Check sheet for the modelled part. Datum: model origin and axes. Units: mm. Face numbers are marked on the shaded views. Coordinates: 2 decimals unless noted, no trailing zeros. Order: outer loops, then holes, each group sorted by start corner. A loop starts at its lowest first (then second) coordinate and runs counter-clockwise, first axis right, second up.
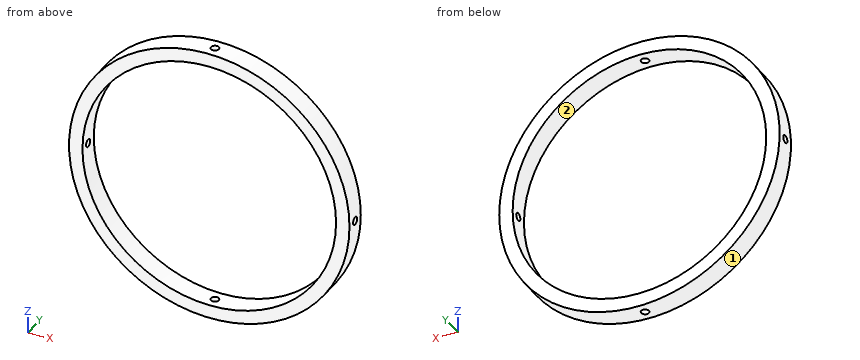
from build123d import *

# Parameters (mm, degrees)
SKETCH1_R               = 52.25
SKETCH1_R_2             = 47.25
BOSS_EXTRUDE1_DEPTH     = 8
SKETCH2_R               = 1.45
CUT_EXTRUDE1_DEPTH      = 53.25
CUT_EXTRUDE1_DEPTH_BACK = 53.25
SKETCH3_R               = 1.45
CUT_EXTRUDE2_DEPTH      = 53.2500001
CUT_EXTRUDE2_DEPTH_BACK = 53.2500001


with BuildPart() as part:
    # Sketch1 → Boss-Extrude1 (new body)
    with BuildSketch(Plane(origin=(0, 0, 0), x_dir=(1, 0, 0), z_dir=(0, 1, 0))):
        Circle(SKETCH1_R)
        Circle(SKETCH1_R_2, mode=Mode.SUBTRACT)
    extrude(amount=BOSS_EXTRUDE1_DEPTH)

    # Sketch2 → Cut-Extrude1 (cut, two sides)
    with BuildSketch(Plane.XY) as cut_extrude1_sk:
        with Locations((0, 4)):
            Circle(SKETCH2_R)
    extrude(amount=CUT_EXTRUDE1_DEPTH, mode=Mode.SUBTRACT)
    extrude(cut_extrude1_sk.sketch, amount=-CUT_EXTRUDE1_DEPTH_BACK, mode=Mode.SUBTRACT)

    # Sketch3 → Cut-Extrude2 (cut, two sides)
    with BuildSketch(Plane(origin=(0, 0, 0), x_dir=(0, 0, -1), z_dir=(1, 0, 0))) as cut_extrude2_sk:
        with Locations((0, 4)):
            Circle(SKETCH3_R)
    extrude(amount=CUT_EXTRUDE2_DEPTH, mode=Mode.SUBTRACT)
    extrude(cut_extrude2_sk.sketch, amount=-CUT_EXTRUDE2_DEPTH_BACK, mode=Mode.SUBTRACT)


solid = part.part
(1) Cross-section at C-C (z = 40). Enter the section's corners in (x, y), and give its area (3 significant figures).
Filled in:
outline: (-33.62, 0) - (-25.15, 0) - (-25.15, 8) - (-33.62, 8) - close; (25.15, 0) - (33.62, 0) - (33.62, 8) - (25.15, 8) - close
area: 135 mm2
(2) Cross-section at D-D (y = 1.25). Enter the section's corners in (x, z).
Filled in:
outline: circle Ø104.5 at (0, 0); hole circle Ø94.5 at (0, 0)
(3) Release check for a two-part mould opening along Z. For the marked faces 1 and 2 record: +Z half, -Z half, draft (parallel to the pull), parting line (faces both ways), or undercut.
Filled in:
face 1: parting line
face 2: undercut
(4) Cross-section at A-A (x = 0). Enter the section's corners in (y, z).
Filled in:
outline: (0, -52.25) - (2.55, -52.25) - (2.55, -47.25) - (0, -47.25) - close; (0, 47.25) - (2.55, 47.25) - (2.55, 52.25) - (0, 52.25) - close; (5.45, -52.25) - (8, -52.25) - (8, -47.25) - (5.45, -47.25) - close; (5.45, 47.25) - (8, 47.25) - (8, 52.25) - (5.45, 52.25) - close
(5) Cross-section at B-B (x = -24.5). Enter the section's corners in (y, z), and give its area (3 significant figures).
Filled in:
outline: (0, -46.15) - (8, -46.15) - (8, -40.4) - (0, -40.4) - close; (0, 40.4) - (8, 40.4) - (8, 46.15) - (0, 46.15) - close
area: 92.0 mm2
(6) Thickness scan on probe 1 along Z at (x, y) = (1.5, 7.5); probe 2 along X at (y, z) = (2.25, 0); probe 3 along Y at (x, z) = (49.3, 0). Record the ranges inside material, lowest first.
Filled in:
probe 1: z = -52.23 to -47.23, 47.23 to 52.23
probe 2: x = -52.25 to -47.25, 47.25 to 52.25
probe 3: y = 0 to 2.55, 5.45 to 8
(7) Go/stop test with flat-tipped pins: P1, Ø2, axis at x = -15, y = 3.5, coming from the +Z side; P2, Ø1.5, axis at y = 2.5, z = 35, coming from the +X side; P3, Ø2, axis at y = 6.5, z = 31.5, coming from the +X side. Record where each tip stops, or that it passes through.
Filled in:
P1: stops at z = 50.34
P2: stops at x = 39.46
P3: stops at x = 42.42
